Part model, mm, in its own coordinate system. Face numbers are marked on the shaded views. A direction names the side the tool comes from. Give positions to 0.01 mm unless a question says otherwise; leave off trailing zeros. Loops run counter-clockwise (first coordinate to the right, second up) from the corner with the lowest first, then second, coordinate; pieces in that order, holes last. Notation, with made-up numbers: (73.25, -36.75) -> (77.25, -36.75) arc R21 cw to (77.25, -8.75) -> close; hole circle Ø5 at (-38, 30). An arc over 180 degrees is marked (long way). One line per question, with ' | ' between items.
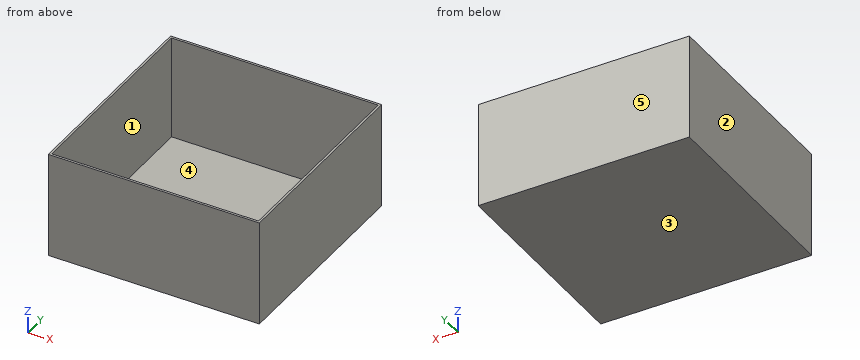
```python
from build123d import *

# Parameters (mm, degrees)
SKETCH1_W           = 152.4
SKETCH1_H           = 152.4
BOSS_EXTRUDE1_DEPTH = 76.2
SHELL1_T            = -1.5875


with BuildPart() as part:
    # Sketch1 → Boss-Extrude1 (new body)
    with BuildSketch(Plane.XY):
        with Locations((76.2, 76.2)):
            Rectangle(SKETCH1_W, SKETCH1_H)
    extrude(amount=BOSS_EXTRUDE1_DEPTH)

    # Shell1
    shell1_openings = [part.faces().sort_by_distance(p)[0] for p in [
        (76.2, 76.2, 76.2),
    ]]
    offset(amount=SHELL1_T, openings=shell1_openings, kind=Kind.INTERSECTION)


solid = part.part
```
1) Tool access for the marked faces 4 and 5: list every direction of +Z, -Z, +X, -X, +Y, -Y with a clear straight run to the whole face (end or side of a thin tool).
Found:
face 4: +Z | face 5: +Z, -Z, +X, -X, +Y
2) Pull direction X, two halves, no side cores. Call the marked faces 1, 2 and 3: pulls with the +X half, pulls with the -X half, needs draft (parallel to the pull), parting line crosses it, or undercut.
Found:
face 1: undercut | face 2: pulls with the -X half | face 3: needs draft
3) Drill centre lines: line 1 (X direction, y = 97.5, z = 43.5); line 2 (Z direction, x = 13, y = 73.5). Where is each one in solid material? Low to high.
Found:
line 1: 0 to 1.59, 150.81 to 152.4 | line 2: 0 to 1.59
4) Saw through at A-A (z = 36). Give the cut face in (x, y).
Found:
outline: (0, 0) -> (152.4, 0) -> (152.4, 152.4) -> (0, 152.4) -> close; hole (1.59, 1.59) -> (150.81, 1.59) -> (150.81, 150.81) -> (1.59, 150.81) -> close
5) Pin check, flat tips, straight feed: P1, Ø22.5, axis at x = 76.5, z = 36, coming from the -Y side; P2, Ø1.5, axis at x = 80.5, y = 65.5, coming from the +Z side. Stop position of each tip, or through.
Found:
P1: y = 0 | P2: z = 1.59
6) Saw through at B-B (x = 83.5). Give the cut face in (y, z), and give its area (3 significant figures).
Found:
outline: (0, 0) -> (152.4, 0) -> (152.4, 76.2) -> (150.81, 76.2) -> (150.81, 1.59) -> (1.59, 1.59) -> (1.59, 76.2) -> (0, 76.2) -> close | area: 479 mm2
